from build123d import *

# Parameters (mm, degrees)
SKETCH_1_W               = 80
SKETCH_1_H               = 35
EXTRUDE_1_DEPTH          = 2
SKETCH_2_R               = 2.5
EXTRUDE_2_DEPTH          = 5
SKETCH_3_R               = 1.25
CUT_EXTRUDE_1_DEPTH      = 1
CUT_EXTRUDE_1_DEPTH_BACK = 8
FILLET_1_R               = 2
FILLET_2_R               = 2
FILLET_3_R               = 2
FILLET_4_R               = 2
SKETCH_5_R               = 1.25
CUT_EXTRUDE_3_DEPTH      = 10
SKETCH_6_R               = 2.5
SKETCH_6_R_2             = 1.25
EXTRUDE_3_DEPTH          = 4
SKETCH_7_W               = 49.218742156
SKETCH_7_H               = 20
SKETCH_7_R               = 2.25
EXTRUDE_4_DEPTH          = 2


with BuildPart() as part:
    # Эскиз1 → Бобышка-Вытянуть1 (new body)
    with BuildSketch(Plane(origin=(0, 0, 0), x_dir=(1, 0, 0), z_dir=(0, 1, 0))):
        with Locations((40, -17.5)):
            Rectangle(SKETCH_1_W, SKETCH_1_H)
    extrude(amount=EXTRUDE_1_DEPTH)

    # Эскиз2 → Бобышка-Вытянуть2 (add)
    with BuildSketch(Plane(origin=(0, 2, 0), x_dir=(1, 0, 0), z_dir=(0, 1, 0))):
        with Locations((11, -6)):
            Circle(SKETCH_2_R)
        with Locations((11, -29)):
            Circle(SKETCH_2_R)
        with Locations((69, -6)):
            Circle(SKETCH_2_R)
        with Locations((69, -29)):
            Circle(SKETCH_2_R)
    extrude(amount=EXTRUDE_2_DEPTH)

    # Эскиз3 → Вырез-Вытянуть1 (cut, two sides)
    with BuildSketch(Plane(origin=(0, 7, 0), x_dir=(1, 0, 0), z_dir=(0, 1, 0))) as cut_extrude_1_sk:
        with Locations((11, -6)):
            Circle(SKETCH_3_R)
        with Locations((11, -29)):
            Circle(SKETCH_3_R)
        with Locations((69, -6)):
            Circle(SKETCH_3_R)
        with Locations((69, -29)):
            Circle(SKETCH_3_R)
    extrude(amount=CUT_EXTRUDE_1_DEPTH, mode=Mode.SUBTRACT)
    extrude(cut_extrude_1_sk.sketch, amount=-CUT_EXTRUDE_1_DEPTH_BACK, mode=Mode.SUBTRACT)

    # Скругление1
    fillet_1_edges = [part.edges().sort_by_distance(p)[0] for p in [
        (0, 1, 0),
    ]]
    fillet(fillet_1_edges, radius=FILLET_1_R)

    # Скругление2
    fillet_2_edges = [part.edges().sort_by_distance(p)[0] for p in [
        (0, 1, 35),
    ]]
    fillet(fillet_2_edges, radius=FILLET_2_R)

    # Скругление3
    fillet_3_edges = [part.edges().sort_by_distance(p)[0] for p in [
        (80, 1, 35),
    ]]
    fillet(fillet_3_edges, radius=FILLET_3_R)

    # Скругление4
    fillet_4_edges = [part.edges().sort_by_distance(p)[0] for p in [
        (80, 1, 0),
    ]]
    fillet(fillet_4_edges, radius=FILLET_4_R)

    # Эскиз5 → Вырез-Вытянуть3 (cut)
    with BuildSketch(Plane.XZ):
        with Locations((16.789329721, 26.745983075)):
            Circle(SKETCH_5_R)
        with Locations((72.789329721, 26.745983075)):
            Circle(SKETCH_5_R)
        with Locations((72.789329721, 7.745983075)):
            Circle(SKETCH_5_R)
        with Locations((16.789329721, 7.745983075)):
            Circle(SKETCH_5_R)
    extrude(amount=-CUT_EXTRUDE_3_DEPTH, mode=Mode.SUBTRACT)

    # Эскиз6 → Бобышка-Вытянуть3 (add)
    with BuildSketch(Plane.XZ):
        with Locations((16.789329721, 26.745983075)):
            Circle(SKETCH_6_R)
        with Locations((16.789329721, 26.745983075)):
            Circle(SKETCH_6_R_2, mode=Mode.SUBTRACT)
        with Locations((72.789329721, 26.745983075)):
            Circle(SKETCH_6_R)
        with Locations((72.789329721, 26.745983075)):
            Circle(SKETCH_6_R_2, mode=Mode.SUBTRACT)
        with Locations((72.789329721, 7.745983075)):
            Circle(SKETCH_6_R)
        with Locations((72.789329721, 7.745983075)):
            Circle(SKETCH_6_R_2, mode=Mode.SUBTRACT)
        with Locations((16.789329721, 7.745983075)):
            Circle(SKETCH_6_R)
        with Locations((16.789329721, 7.745983075)):
            Circle(SKETCH_6_R_2, mode=Mode.SUBTRACT)
    extrude(amount=EXTRUDE_3_DEPTH)

    # Эскиз7 → Бобышка-Вытянуть4 (add)
    with BuildSketch(Plane.ZY):
        with Locations((17.5, 1)):
            Rectangle(SKETCH_7_W, SKETCH_7_H)
        with Locations((38.109371078, -5)):
            Circle(SKETCH_7_R, mode=Mode.SUBTRACT)
        with Locations((-3.109371078, -5)):
            Circle(SKETCH_7_R, mode=Mode.SUBTRACT)
        with Locations((-3.109371078, 7)):
            Circle(SKETCH_7_R, mode=Mode.SUBTRACT)
        with Locations((38.109371078, 7)):
            Circle(SKETCH_7_R, mode=Mode.SUBTRACT)
    extrude(amount=-EXTRUDE_4_DEPTH)


solid = part.part
Model file for the job. Use its own axes, mm. A direction names the side the tool comes from. Give positions to 0.01 mm unless a question says otherwise; leave off trailing zeros. Write each loop counter-clockwise with the first axis right and the second up, starting at its lowest first coordinate (ties: lowest second). Pieces come first, ordered by that corner, then holes. Notation, with made-up numbers: M 30,52 L 62,52 A28 ccw 62,71 Z; hole C 85,-15.5 d10. An arc over 180 degrees is marked long. One line per item, written item: value. Start each with the question number.
Q1. Two-plate mould, pull along X, no slides. Class faces 1 (the cylindrical face through (75.174, -1.972, 27.497)), 2 (the flat face through (80, 1, 18)), 3 (the cylindrical face through (19.1, -1.97, 6.79)), 4 (the flat face through (1, 1, -7.109)): +X half, -X half, draft (parallel to the pull), parting line (faces both ways), or undercut.
Q2. Saw through at A-A, the plane x = 11. Write the cut outline in (y, z).
Q3. Saw through at B-B, the plane y = -5. Write the cut outline in (x, z), plus the area to 3 significant figures.
Q4. Drop flat-ended pins along their axis: pin 1 Ø3 at (y, z) = (-6.5, 18.5) entering from -X; pin 2 Ø5.5 at (x, z) = (15.5, 8.5) entering from -Y; pin 3 Ø4 at (x, z) = (52, 2) entering from +Y; pin 4 Ø1 at (x, z) = (70, 9.5) entering from -Y. Give the stop position or say it passes through.
Q5. Saw through at C-C, the plane x = 51. Write the cut outline in (y, z).
Q6. 3-axis set-ups, long thin cutter, end or side, ignore diameter. For faces 5 (the flat face through (72, -4, 9)), 6 (the flat face through (10, 7, 7)), 7 (the cylindrical face through (9.16, 4.46, 4.31)), 8 (the flat face through (39, 1, 35)): which of +Z, -Z, +X, -X, +Y, -Y reach the whole face in a straight line?
Q7. Probe probe 1 along X at (y, z) = (1.5, 29); probe 2 along Z at (x, y) = (11, 4.25); probe 3 along X at (y, z) = (-3.75, 6). List the from-to ranges inside material, lowest first. Write a range as [from, to].
Output values:
1. face 1: undercut
1. face 2: +X half
1. face 3: undercut
1. face 4: draft
2. outline: M 0,0 L 2,0 L 2,3.5 L 7,3.5 L 7,4.75 L 0,4.75 Z; M 0,7.25 L 7,7.25 L 7,8.5 L 2,8.5 L 2,26.5 L 7,26.5 L 7,27.75 L 0,27.75 Z; M 0,30.25 L 7,30.25 L 7,31.5 L 2,31.5 L 2,35 L 0,35 Z
3. outline: M 0,-7.11 L 2,-7.11 L 2,-5.36 L 0,-5.36 Z; M 0,-0.86 L 2,-0.86 L 2,35.86 L 0,35.86 Z; M 0,40.36 L 2,40.36 L 2,42.11 L 0,42.11 Z
3. area: 80.4 mm²
4. pin 1: stops at x = 0
4. pin 2: stops at y = -4
4. pin 3: stops at y = 2
4. pin 4: stops at y = 0
5. outline: M 0,0 L 2,0 L 2,35 L 0,35 Z
6. face 5: +Z, -Z, +X, -Y
6. face 6: +Z, -Z, +X, +Y
6. face 7: +Y
6. face 8: +Z, +X, +Y, -Y
7. probe 1: x = [0, 9.75], [12.25, 67.75], [70.25, 80]
7. probe 2: z = [3.5, 4.75], [7.25, 8.5], [26.5, 27.75], [30.25, 31.5]
7. probe 3: x = [0, 2], [15, 18.58], [71, 74.58]
